Build history of the part. All positions in model axes, mm. A direction names the side the tool comes from. Round coordinates to 2 decimals unless told otherwise and drop trailing zeros. Write each loop counter-clockwise with the first axis right and the second up, starting at its lowest first coordinate (ties: lowest second). Pieces come first, ordered by that corner, then holes. Notation, with made-up numbers: M -34.75,29 L 23.25,29 A15 cw 23.25,42 Z; hole C 40.5,-22 d6. An arc over 180 degrees is marked long. Write item = value, one per line. Start each with the question number.
Q1. Tool access for faces 4 (the flat face through (-2, 22.225, 3)), 5 (the cylindrical face through (4.77, -14.75, 1.57)): list every direction of +Z, -Z, +X, -X, +Y, -Y with a clear straight run to the whole face (end or side of a thin tool).
Q2. Pull direction X, two halves, no side cores. Call faces 1 (the flat face through (-2, 0, 0)), 2 (the flat face through (115.888, 0, 3)), 3 (the cylindrical face through (4.83, -3.565, 1.565)): released by +X, released by -X, zero draft, split by the parting line, or undercut.
Q3. Band-saw the part on B-B on z = 2. Write the cut outline in (x, y) (1 decimal), plus the area to 3 significant figures.
Q4. Band-saw the part on A-A on x = 88.9. Write the cut outline in (y, z) (3 decimals), plus the area to 3 significant figures.
Q5. Probe L1, parallel to Y at x = -15, z = 0.5 (3 decimals); L2, parallel to X at y = -7, z = 2.25; L3, parallel to Y at x = 88.9, z = 5.25 (3 decimals). List the from-to ranges inside material, lowest first.
Q6. Band-saw the part on C-C on x = -85.5. Write the cut outline in (y, z) (3 decimals), plus the area to 3 significant figures.
Q7. Drop a flat-ended pin along its axis: P1, Ø6, axis at x = 49.5, y = -6, coming from the -Z side (3 decimals). Give the stop position or say it passes through.
```python
from build123d import *

# Parameters (mm, degrees)
SKETCH1_W           = 231.775
SKETCH1_H           = 44.45
BOSS_EXTRUDE1_DEPTH = 6.35
CUT_EXTRUDE1_REACH  = 120.17
SKETCH2_R           = 12.7
SKETCH2_W           = 13.49375
SKETCH2_H           = 7.14375
SKETCH2_W_2         = 26.19375
SKETCH2_H_2         = 5.30225
FILLET1_R           = 0.762
CUT_EXTRUDE2_DEPTH  = 3.175
CUT_EXTRUDE3_DEPTH  = 3.175


with BuildPart() as part:
    # Sketch1 → Boss-Extrude1 (new body)
    with BuildSketch(Plane.XY):
        Rectangle(SKETCH1_W, SKETCH1_H)
    extrude(amount=BOSS_EXTRUDE1_DEPTH)

    # Sketch2 → Cut-Extrude1 (cut, up to next)
    with BuildSketch(Plane.XY.offset(6.35), mode=Mode.PRIVATE) as cut_extrude1_sk1:
        with Locations((88.9, -3.175)):
            Circle(SKETCH2_R)
    cut_extrude1_tool1 = extrude(cut_extrude1_sk1.sketch, amount=-CUT_EXTRUDE1_REACH, mode=Mode.PRIVATE) & part.part
    # Sketch2 → Cut-Extrude1 (cut, up to next)
    with BuildSketch(Plane.XY.offset(6.35), mode=Mode.PRIVATE) as cut_extrude1_sk2:
        with Locations((-88.9, -3.175)):
            Circle(SKETCH2_R)
    cut_extrude1_tool2 = extrude(cut_extrude1_sk2.sketch, amount=-CUT_EXTRUDE1_REACH, mode=Mode.PRIVATE) & part.part
    # Sketch2 → Cut-Extrude1 (cut, up to next)
    with BuildSketch(Plane.XY.offset(6.35), mode=Mode.PRIVATE) as cut_extrude1_sk3:
        with Locations((-22.225, -9.128125)):
            Rectangle(SKETCH2_W, SKETCH2_H)
    cut_extrude1_tool3 = extrude(cut_extrude1_sk3.sketch, amount=-CUT_EXTRUDE1_REACH, mode=Mode.PRIVATE) & part.part
    # Sketch2 → Cut-Extrude1 (cut, up to next)
    with BuildSketch(Plane.XY.offset(6.35), mode=Mode.PRIVATE) as cut_extrude1_sk4:
        with Locations((-3.96875, -9.128125)):
            Rectangle(SKETCH2_W, SKETCH2_H)
    cut_extrude1_tool4 = extrude(cut_extrude1_sk4.sketch, amount=-CUT_EXTRUDE1_REACH, mode=Mode.PRIVATE) & part.part
    # Sketch2 → Cut-Extrude1 (cut, up to next)
    with BuildSketch(Plane.XY.offset(6.35), mode=Mode.PRIVATE) as cut_extrude1_sk5:
        with Locations((52.3875, -5.826125)):
            Rectangle(SKETCH2_W_2, SKETCH2_H_2)
    cut_extrude1_tool5 = extrude(cut_extrude1_sk5.sketch, amount=-CUT_EXTRUDE1_REACH, mode=Mode.PRIVATE) & part.part
    add(cut_extrude1_tool1.solids().sort_by_distance((88.9, -3.175, 6.35))[0], mode=Mode.SUBTRACT)
    add(cut_extrude1_tool2.solids().sort_by_distance((-88.9, -3.175, 6.35))[0], mode=Mode.SUBTRACT)
    add(cut_extrude1_tool3.solids().sort_by_distance((-22.225, -9.128125, 6.35))[0], mode=Mode.SUBTRACT)
    add(cut_extrude1_tool4.solids().sort_by_distance((-3.96875, -9.128125, 6.35))[0], mode=Mode.SUBTRACT)
    add(cut_extrude1_tool5.solids().sort_by_distance((52.3875, -5.826125, 6.35))[0], mode=Mode.SUBTRACT)

    # Fillet1
    fillet1_edges = [part.edges().sort_by_distance(p)[0] for p in [
        (-28.971875, -5.55625, 3.175),
        (-15.478125, -5.55625, 3.175),
        (-15.478125, -12.7, 3.175),
        (-28.971875, -12.7, 3.175),
        (-10.715625, -12.7, 3.175),
        (-10.715625, -5.55625, 3.175),
        (2.778125, -5.55625, 3.175),
        (2.778125, -12.7, 3.175),
        (39.290625, -8.47725, 3.175),
        (39.290625, -3.175, 3.175),
        (65.484375, -3.175, 3.175),
        (65.484375, -8.47725, 3.175),
    ]]
    fillet(fillet1_edges, radius=FILLET1_R)

    # Sketch3 → Cut-Extrude2 (cut)
    with BuildSketch(Plane(origin=(0, 0, 0), x_dir=(-1, 0, 0), z_dir=(0, 0, -1))):
        with BuildLine():
            Line((-64.722375, -11.65225), (-40.052625, -11.65225))
            ThreePointArc((-40.052625, -11.65225), (-37.268745602, -10.499129398), (-36.115625, -7.71525))
            Line((-36.115625, -7.71525), (-36.115625, -3.937))
            ThreePointArc((-36.115625, -3.937), (-37.268745602, -1.153120602), (-40.052625, 0))
            Line((-40.052625, 0), (-64.722375, 0))
            ThreePointArc((-64.722375, 0), (-67.506254398, -1.153120602), (-68.659375, -3.937))
            Line((-68.659375, -3.937), (-68.659375, -7.71525))
            ThreePointArc((-68.659375, -7.71525), (-67.506254398, -10.499129398), (-64.722375, -11.65225))
        make_face()
    extrude(amount=-CUT_EXTRUDE2_DEPTH, mode=Mode.SUBTRACT)

    # Sketch4 → Cut-Extrude3 (cut)
    with BuildSketch(Plane(origin=(0, 0, 0), x_dir=(-1, 0, 0), z_dir=(0, 0, -1))):
        with BuildLine():
            Line((28.209875, -15.875), (-2.016125, -15.875))
            ThreePointArc((-2.016125, -15.875), (-4.800004398, -14.721879398), (-5.953125, -11.938))
            Line((-5.953125, -11.938), (-5.953125, -6.31825))
            ThreePointArc((-5.953125, -6.31825), (-4.800004398, -3.534370602), (-2.016125, -2.38125))
            Line((-2.016125, -2.38125), (28.209875, -2.38125))
            ThreePointArc((28.209875, -2.38125), (30.993754398, -3.534370602), (32.146875, -6.31825))
            Line((32.146875, -6.31825), (32.146875, -11.938))
            ThreePointArc((32.146875, -11.938), (30.993754398, -14.721879398), (28.209875, -15.875))
        make_face()
    extrude(amount=-CUT_EXTRUDE3_DEPTH, mode=Mode.SUBTRACT)


solid = part.part
```
Conclusion:
q1.face_4 = +Z, -Z, +X, -X, +Y
q1.face_5 = -Z
q2.face_1 = zero draft
q2.face_2 = released by +X
q2.face_3 = undercut
q3.outline = M -115.9,-22.2 L 115.9,-22.2 L 115.9,22.2 L -115.9,22.2 Z; hole C -88.9,-3.2 d25.4; hole M -32.1,-11.9 A3.9 ccw -28.2,-15.9 L 2,-15.9 A3.9 ccw 6,-11.9 L 6,-6.3 A3.9 ccw 2,-2.4 L -28.2,-2.4 A3.9 ccw -32.1,-6.3 Z; hole M 36.1,-7.7 A3.9 ccw 40.1,-11.7 L 64.7,-11.7 A3.9 ccw 68.7,-7.7 L 68.7,-3.9 A3.9 ccw 64.7,0 L 40.1,0 A3.9 ccw 36.1,-3.9 Z; hole C 88.9,-3.2 d25.4
q3.area = 8,420 mm^2
q4.outline = M -22.225,0 L -15.875,0 L -15.875,6.35 L -22.225,6.35 Z; M 9.525,0 L 22.225,0 L 22.225,6.35 L 9.525,6.35 Z
q4.area = 121 mm^2
q5.L1 = -22.225 to -15.875, -2.381 to 22.225
q5.L2 = -115.89 to -101.01, -76.79 to -32.15, 5.95 to 36.12, 68.66 to 76.79, 101.01 to 115.89
q5.L3 = -22.225 to -15.875, 9.525 to 22.225
q6.outline = M -22.225,0 L -15.411,0 L -15.411,6.35 L -22.225,6.35 Z; M 9.061,0 L 22.225,0 L 22.225,6.35 L 9.061,6.35 Z
q6.area = 127 mm^2
q7.P1 = 3.175
